The listing builds one solid part. Answer for the finished solid, in the listing's coordinates (mm). A direction names the side the tool comes from. Coordinates: 2 decimals unless noted, no trailing zeros. Loops run counter-clockwise (first coordinate to the right, second up) from the corner with the lowest first, then second, coordinate; pieces in that order, holes last. Notation, with made-up numbers: (17.25, 46) - (21.25, 46) arc R32 cw to (21.25, 83) - close; hole circle Ø5 at (45, -18). An arc over 180 degrees is marked (long way). Return JSON: item names as keys, results as strings. Group by question number.
1. Section D-D (y = -17) is taken. Write down the section's boundary in (x, z).
2. Section B-B (x = 17) is taken. Write down the section's boundary in (y, z).
3. Find the intervals of material crossed by line 1 along Z through (x, y) = (1.5, 16); line 2 along Z through (x, y) = (-15, -11.5); line 3 along Z through (x, y) = (8.5, 8.5), in increasing order.
4. The mould has two halves that part along X. Classify faces 6 (the face through (0, 0, 9)), 7 (the face through (23.846, 7.509, 1.479)), 8 (the face through (12.89, 13.49, -15.46)), 9 (the face through (-13.06, 13.95, -15.46)): pulls with the +X half, pulls with the -X half, needs draft (parallel to the pull), parting line crosses it, or undercut.
5. Section A-A (y = 22.5) is taken. Write down the section's boundary in (x, z), and give its area (3 significant figures).
6. Which of the six approach directions +Z, -Z, +X, -X, +Y, -Y give full straight-line access (tool end or side, diameter ignored) to faces 1 (the face through (23.846, 7.509, -11.479)), 2 (the face through (0, 0, -19)), 3 (the face through (-6, -7, -13)), 4 (the face through (-0.1, -7.5, 6)), 5 (the face through (12.89, 13.49, 5.97))?
7. Section C-C (z = -8) is taken. Write down the section's boundary in (x, y).
8. Each of these flat-tipped pins is pushed along its axis until it touches: P1, Ø6, axis at x = 2, y = -1.5, coming from the -Z side; P2, Ø8, axis at x = -17.5, z = -9.5, coming from the -Y side; P3, Ø6, axis at x = 13, z = -14, coming from the -Y side; P4, Ø10, axis at x = 18.5, y = 28.5, coming from the +Z side. Where does it stop, or does it pass through?
```python
from build123d import *

# Parameters (mm, degrees)
SKETCH_1_R          = 25
EXTRUDE_1_DEPTH     = 3
SKETCH_2_R          = 4
EXTRUDE_2_DEPTH     = 5
SKETCH_3_R          = 3.9
EXTRUDE_4_DEPTH     = 6
SKETCH_5_R          = 15
EXTRUDE_5_DEPTH     = 10
EXTRUDE_START       = 6
SKETCH_6_R          = 3.9
EXTRUDE_6_DEPTH     = 6
SKETCH_8_W          = 50
SKETCH_8_H          = 40
EXTRUDE_7_DEPTH     = 5
SKETCH_2_3_R        = 4
CUT_EXTRUDE_1_DEPTH = 1


with BuildPart() as part:
    # Sketch 1 → Extrude 1 (new body)
    with BuildSketch(Plane.XY):
        Circle(SKETCH_1_R)
    extrude_1 = extrude(amount=EXTRUDE_1_DEPTH)

    # Sketch 2 → Extrude 2 (add)
    with BuildSketch(Plane.XY.offset(3)):
        with BuildLine():
            Line((-18.900440322, 30), (-7.047694656, -2.565151075))
            ThreePointArc((-7.047694656, -2.565151075), (0, -7.5), (7.047694656, -2.565151075))
            Line((7.047694656, -2.565151075), (18.900440322, 30))
            Line((18.900440322, 30), (-18.900440322, 30))
        make_face()
        Circle(SKETCH_2_R, mode=Mode.SUBTRACT)
    extrude_2 = extrude(amount=EXTRUDE_2_DEPTH)

    # Sketch 3 → Extrude 4 (add)
    with BuildSketch(Plane.XY.offset(3)):
        Circle(SKETCH_3_R)
    extrude(amount=EXTRUDE_4_DEPTH)

    # Sketch 5 → Extrude 5 (add)
    with BuildSketch(Plane(origin=(0, 0, 0), x_dir=(-1, 0, 0), z_dir=(0, 0, -1))):
        Circle(SKETCH_5_R)
    extrude(amount=EXTRUDE_5_DEPTH)

    # Mirror 1: Extrude 1, Extrude 2 across plane
    add(extrude_1.mirror(Plane.XY.offset(-5)))
    add(extrude_2.mirror(Plane.XY.offset(-5)))

    # Sketch 6 → Extrude 6 (add)
    with BuildSketch(Plane(origin=(0, 0, -13), x_dir=(-1, 0, 0), z_dir=(0, 0, -1)).offset(EXTRUDE_START)):
        with Locations(Location((0, 0, 0), (0, 0, 180))):
            Circle(SKETCH_6_R)
    extrude(amount=-EXTRUDE_6_DEPTH)

    # Sketch 8 → Extrude 7 (add)
    with BuildSketch(Plane(origin=(0, 30, 0), x_dir=(1, 0, 0), z_dir=(0, 1, 0))):
        with Locations((0, 10)):
            Rectangle(SKETCH_8_W, SKETCH_8_H)
    extrude(amount=EXTRUDE_7_DEPTH)

    # Sketch 2_3 → Cut-Extrude 1 (cut)
    with BuildSketch(Plane.XY.offset(3)):
        with BuildLine():
            Line((-18.900440322, 30), (-7.047694656, -2.565151075))
            ThreePointArc((-7.047694656, -2.565151075), (0, -7.5), (7.047694656, -2.565151075))
            Line((7.047694656, -2.565151075), (18.900440322, 30))
            Line((18.900440322, 30), (-18.900440322, 30))
        make_face()
        Circle(SKETCH_2_3_R, mode=Mode.SUBTRACT)
    extrude(amount=CUT_EXTRUDE_1_DEPTH, mode=Mode.SUBTRACT)


solid = part.part
```
The answers:
{
 "1": {"outline": "(-18.33, -13) - (18.33, -13) - (18.33, -10) - (-18.33, -10) - close; (-18.33, 0) - (18.33, 0) - (18.33, 3) - (-18.33, 3) - close"},
 "2": {"outline": "(-18.33, -13) - (18.33, -13) - (18.33, -10) - (-18.33, -10) - close; (-18.33, 0) - (18.33, 0) - (18.33, 3) - (-18.33, 3) - close; (24.78, -18) - (30, -18) - (30, -30) - (35, -30) - (35, 10) - (30, 10) - (30, 8) - (24.78, 8) - (24.78, 4) - (30, 4) - (30, -13) - (24.78, -13) - close"},
 "3": {"line 1": "z = -18 to -10, 0 to 3, 4 to 8", "line 2": "z = -13 to -10, 0 to 3", "line 3": "z = -18 to 3, 4 to 8"},
 "4": {"face 6": "needs draft", "face 7": "parting line crosses it", "face 8": "pulls with the +X half", "face 9": "pulls with the -X half"},
 "5": {"outline": "(-16.17, -18) - (16.17, -18) - (16.17, -13) - (10.9, -13) - (10.9, -10) - (-10.9, -10) - (-10.9, -13) - (-16.17, -13) - close; (-16.17, 4) - (16.17, 4) - (16.17, 8) - (-16.17, 8) - close; (-10.9, 0) - (10.9, 0) - (10.9, 3) - (-10.9, 3) - close", "area": "422 mm2"},
 "6": {"face 1": "none", "face 2": "-Z, +X, -X, -Y", "face 3": "-Z, -Y", "face 4": "+Z, -Y", "face 5": "+Z, +X, -Y"},
 "7": {"outline": "(-25, 30) - (25, 30) - (25, 35) - (-25, 35) - close; circle Ø30 at (0, 0)"},
 "8": {"P1": "stops at z = -19", "P2": "stops at y = -21.02", "P3": "stops at y = -22.84", "P4": "stops at z = 10"}
}
